Drawing for the job (mm, zero at the part's lowest x, y, z). Give positions to 0.01 mm unless a question says otherwise; leave off trailing zeros. Order: outer loops, then holes, each group sorted by start corner. A loop starts at its lowest first (then second) coordinate and runs counter-clockwise, first axis right, second up. Notation, with made-up numbers: (24.5, 42) - (55.5, 42) arc R13 ccw to (55.5, 63) - close; hole circle Ø5 at (57.5, -25.75). An arc over 180 degrees is marked (long way). Use a Markdown table: item, result. Add a question column.
(1) Slice it at B-B (x = 4). Write the cut outline in (y, z).
(2) Slice it at A-A (y = 4.5). Write the cut outline in (x, z).
(3) Mould opens along Y. For the marked faces 1, 2, 3 and 4 say: +Y half, -Y half, draft (parallel to the pull), parting line (faces both ways), or undercut.
(4) Flat gauge pin, fed straight in: pin 1 (1 mm diameter, centred on x = 3, z = 2, fed in from +Y). Where does the tip first touch, or does it go through?
(5) Slice it at D-D (z = 1.9). Write the cut outline in (x, y).
(6) Wall check: line 1 (X direction, y = 4.5, z = 0.95); line 2 (Y direction, x = 4, z = 0.6); line 3 (X direction, y = 3.75, z = 0.25). Give the ranges that are in metal, low to high.
(7) Slice it at C-C (z = 0.5). Write the cut outline in (x, y).
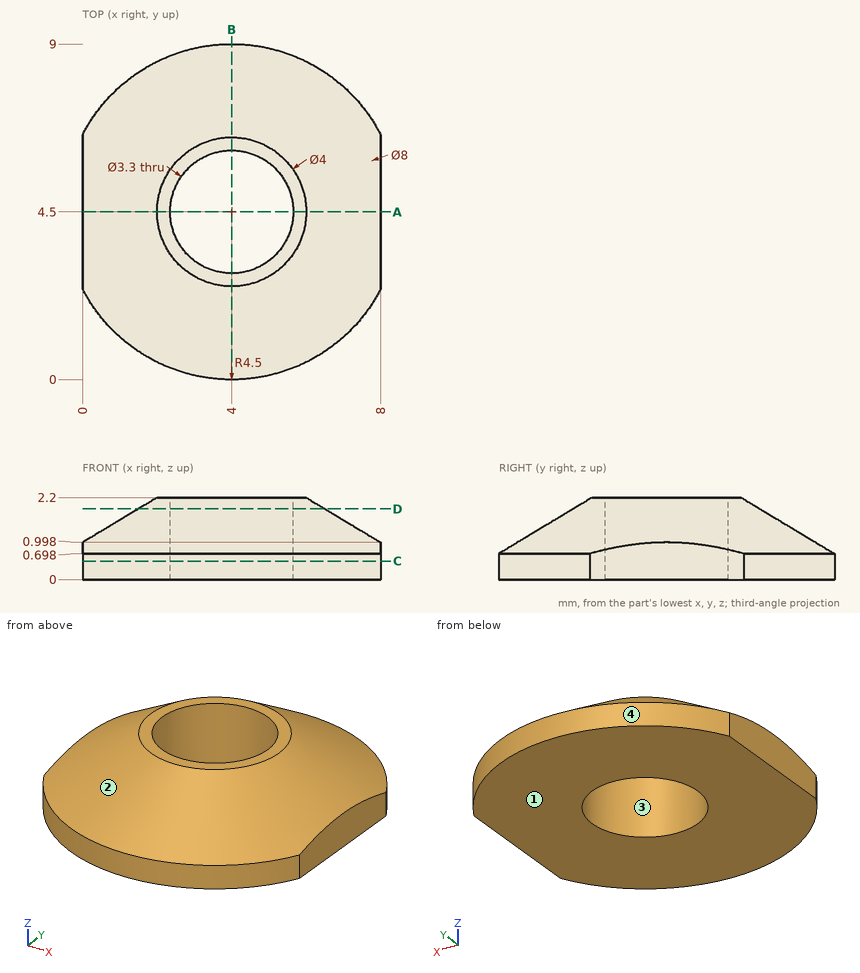
Solution:
| question | item | result |
|---|---|---|
| 1 | outline | (0, 0) - (2.85, 0) - (2.85, 2.2) - (2.5, 2.2) - (0, 0.7) - close; (6.15, 0) - (9, 0) - (9, 0.7) - (6.5, 2.2) - (6.15, 2.2) - close |
| 2 | outline | (0, 0) - (2.35, 0) - (2.35, 2.2) - (2, 2.2) - (0, 1) - close; (5.65, 0) - (8, 0) - (8, 1) - (6, 2.2) - (5.65, 2.2) - close |
| 3 | face 1 | draft |
| 3 | face 2 | parting line |
| 3 | face 3 | undercut |
| 3 | face 4 | +Y half |
| 4 | pin 1 | y = 7.52 |
| 5 | outline | circle Ø5 at (4, 4.5); hole circle Ø3.3 at (4, 4.5) |
| 6 | line 1 | 0 to 2.35, 5.65 to 8 |
| 6 | line 2 | 0 to 2.85, 6.15 to 9 |
| 6 | line 3 | 0 to 2.53, 5.47 to 8 |
| 7 | outline | (0, 2.44) arc R4.5 ccw to (8, 2.44) - (8, 6.56) arc R4.5 ccw to (0, 6.56) - close; hole circle Ø3.3 at (4, 4.5) |
